Geometry check sheet. Reference: the model listing, model coordinates, mm. A direction names the side the tool comes from. Coordinates: 2 decimals unless noted, no trailing zeros. Loops run counter-clockwise (first coordinate to the right, second up) from the corner with the lowest first, then second, coordinate; pieces in that order, holes last.
from build123d import *

# Parameters (mm, degrees)
F0_W     = 100
F0_H     = 50
F1_DEPTH = 100
F3_DEPTH = 85
F4_W     = 15
F4_H     = 50
F5_DEPTH = 25
F7_DEPTH = 15
F9_DEPTH = 50


with BuildPart() as f1:
    # F0 (on Front) → F1 (new body)
    with BuildSketch(Plane.XZ):
        with Locations((50, -25)):
            Rectangle(F0_W, F0_H)
    extrude(amount=F1_DEPTH)

    # F2 (on face) → F3 (cut)
    with BuildSketch(Plane.XZ.offset(100)):
        Polygon((85, 0), (15, 0), (15, -7), (0, -7), (0, -43), (15, -43), (15, -50), (85, -50), (85, -43), (100, -43), (100, -7), (85, -7), align=None)
    extrude(amount=-F3_DEPTH, mode=Mode.SUBTRACT)

    # F4 (on face) → F5 (join)
    with BuildSketch(Plane.XZ.offset(100)):
        with Locations((92.5, -25)):
            Rectangle(F4_W, F4_H)
    extrude(amount=-F5_DEPTH)

    # F6 (on face) → F7 (cut)
    with BuildSketch(Plane.YZ.offset(100)):
        with BuildLine():
            Line((-100, 0), (-100, -50))
            ThreePointArc((-100, -50), (-93.161987, -25), (-100, 0))
        make_face()
    extrude(amount=-F7_DEPTH, mode=Mode.SUBTRACT)

    # F8 (on face) → F9 (cut)
    with BuildSketch(Plane(origin=(0, 0, -50), x_dir=(1, 0, 0), z_dir=(0, 0, -1))):
        with BuildLine():
            Line((15, 100), (0, 100))
            ThreePointArc((0, 100), (7.5, 97.637464), (15, 100))
        make_face()
    extrude(amount=-F9_DEPTH, mode=Mode.SUBTRACT)


solid = f1.part
1) Section check A-A on z = -37. Record the cut outline in (x, y).
Data:
outline: (0, -15) - (100, -15) - (100, 0) - (0, 0) - close; (85, -94.65) - (100, -94.65) - (100, -75) - (85, -75) - close
2) Section check C-C on y = -78. Record the cut outline in (x, z).
Data:
outline: (0, -50) - (15, -50) - (15, -43) - (0, -43) - close; (0, -7) - (15, -7) - (15, 0) - (0, 0) - close; (85, -50) - (100, -50) - (100, 0) - (85, 0) - close
3) Mould release check, pull along X, two halves, no side actions. Record for faces 1 (the flat face through (0, -35, -44)), 2 (the flat face through (49, -15, -25)), 3 (the flat face through (8, -58, -7)), 4 (the flat face through (100, -49, -3)): +X half, -X half, draft (parallel to the pull), parting line (faces both ways), or undercut.
Data:
face 1: -X half
face 2: undercut
face 3: draft
face 4: +X half
4) Section check B-B on y = -22. Record the cut outline in (x, z), and give its area (3 significant figures).
Data:
outline: (0, -50) - (15, -50) - (15, -43) - (0, -43) - close; (0, -7) - (15, -7) - (15, 0) - (0, 0) - close; (85, -50) - (100, -50) - (100, -43) - (85, -43) - close; (85, -7) - (100, -7) - (100, 0) - (85, 0) - close
area: 420 mm2
5) Depth check by flat-ended pin: pin 1 (12 mm diameter, centred on x = 4.5, y = -42, fed in from +Z); pin 2 (10 mm diameter, centred on x = 13, z = -28.5, fed in from -Y); pin 3 (1.5 mm diameter, centred on x = 85, z = -13.5, fed in from -Y). Enter the tip coordinate at first touch or a pass-through.
Data:
pin 1: stops at z = 0
pin 2: stops at y = -15
pin 3: stops at y = -94.71
6) Section check D-D on z = -17.5. Record the cut outline in (x, y), and give its area (3 significant figures).
Data:
outline: (0, -15) - (100, -15) - (100, 0) - (0, 0) - close; (85, -93.74) - (100, -93.74) - (100, -75) - (85, -75) - close
area: 1,780 mm2
7) Material ranges on probe 1 along X at (y, z) = (-89.5, -3); probe 2 along X at (y, z) = (-80.5, -39); probe 3 along Y at (x, z) = (47.5, -21), recorded low to high.
Data:
probe 1: x = 0 to 15, 85 to 100
probe 2: x = 85 to 100
probe 3: y = -15 to 0
8) Access from +Z, -Z, +X, -X, +Y, -Y to the whole of each face (thin tool, end or side, straight path). Record for faces 5 (the cylindrical face through (92.605, -93.163, -25.367)), 6 (the flat face through (7, -58, -43)), 7 (the flat face through (49, 0, -25)), 8 (the flat face through (15, -58, -3)), 9 (the flat face through (93, -45, -7)).
Data:
face 5: +X, -Y
face 6: -X, -Y
face 7: +Z, -Z, +X, -X, +Y
face 8: +Z, -Z, -Y
face 9: +X, -X
